Build history of the part. All positions in model axes, mm. A direction names the side the tool comes from. Round coordinates to 2 decimals unless told otherwise and drop trailing zeros. Loops run counter-clockwise (first coordinate to the right, second up) from the corner with the lowest first, then second, coordinate; pieces in that order, holes last. Notation, with made-up numbers: M 82,6 L 103,6 A27 ccw 103,38 Z; hole C 32.5,18.5 d7. An arc over 180 degrees is marked long. One line per item, written item: value.
Autodesk Inventor part; units mm, degrees
ref_plane "YZ Plane" through (0, 0, 0) normal (1, 0, 0) x (0, 1, 0)
ref_plane "XZ Plane" through (0, 0, 0) normal (0, 1, 0) x (-1, 0, 0)
ref_plane "XY Plane" through (0, 0, 0) normal (0, 0, 1) x (1, 0, 0)
sketch "Sketch1" plane through (0, 0, 0) normal (0, 1, 0) x (-1, 0, 0)
  line L0 (0, 0) -> (23.6236, 0) construction
  line L1 (0, 0) -> (0, -20.0966) construction
  arc A0 (-8, 0) -> (8, 0) centre (0, 0) ccw
  arc A1 (-2.9468, -7.4375) -> (2.9468, -7.4375) centre (0, -8) ccw
  line L2 (0, -11) -> (-8.5189, -11) construction
  circle A2 centre (0, -8) radius 1.35
  line L3 (-8, 0) -> (8, 0)
  arc A3 (8, 0) -> (-8, 0) centre (0, 0) ccw
  arc A4 (2.9468, 7.4375) -> (-2.9468, 7.4375) centre (0, 8) ccw
  line L4 (0, 11) -> (-8.5189, 11) construction
  circle A5 centre (0, 8) radius 1.35
  dimension "d0" = 16
  dimension "d1" = 22
  dimension "d2" = 6
  dimension "d3" = 2.7
extrude "Extrusion1" add sketch "Sketch1" along normal blind 8
extrude "Extrusion2" cut sketch "Sketch1" against normal blind 7 from surface at 8 contours A2 A0 | A0 A2 | A5 A3 | A3 A5
extrude "Extrusion3" add sketch "Sketch1" against normal blind 3.5 contours L3 A0 A2 | A3 A5 L3 | A2 A0 | A3 A5 picked at (0, -7.5415) picked at (0, 7.5415)
chamfer "Chamfer1" distance 1 angle 45 1 edges at (2.9468, -3.5, 7.4375)
properties part number "caster_body"
Item 1: Slice it at B-B, the plane y = 4.25. Give the cut face in (x, z), and give its area (3 significant figures).
Check values:
outline: M -2.95,-7.44 A3 ccw long 2.95,-7.44 A8 ccw 2.95,7.44 A3 ccw long -2.95,7.44 A8 ccw Z; hole C 0,-8 d2.7; hole C 0,8 d2.7
area: 220 mm2
Item 2: Wall check: line 1 along X through (y, z) = (6.25, -8); line 2 along Z through (x, y) = (0.75, 2.25); line 3 along Y through (x, z) = (-1.5, -7.75). Give the ranges that are in metal, low to high.
Check values:
line 1: x = -3 to -1.35, 1.35 to 3
line 2: z = -10.9 to -9.12, -6.88 to 6.88, 9.12 to 10.9
line 3: y = -2.61 to 8
Item 3: Which spindle directions (+Z, -Z, +X, -X, +Y, -Y) get a long thin tool onto all of the face, cutting with end or side? Do faces 1 (the face through (0, -3.5, 0)), 2 (the face through (0, 1, 8)). Say none if no direction does.
Check values:
face 1: +Z, -Z, +X, -X, -Y
face 2: +Y
Item 4: Slice it at C-C, the plane y = -1.75. Give the cut face in (x, z), and give its area (3 significant figures).
Check values:
outline: C 0,0 d16
area: 201 mm2
Item 5: Pull direction X, two halves, no side cores. Call faces 3 (the face through (0, 4, -11)), 4 (the face through (0, 8, 0)), 5 (the face through (0.176, 4.549, -6.661)): pulls with the +X half, pulls with the -X half, needs draft (parallel to the pull), parting line crosses it, or undercut.
Check values:
face 3: parting line crosses it
face 4: needs draft
face 5: undercut
Item 6: Slice it at A-A, the plane x = 0. Give the cut face in (y, z).
Check values:
outline: M -3.5,-7 L -2.5,-8 L 0,-8 L 0,-11 L 8,-11 L 8,-9.35 L 1,-9.35 L 1,-6.65 L 8,-6.65 L 8,6.65 L 1,6.65 L 1,9.35 L 8,9.35 L 8,11 L 0,11 L 0,8 L -2.5,8 L -3.5,7 Z
Item 7: Drop flat-ended pins along their axis: P1, Ø1, axis at x = -1.5, y = 2, coming from the +Z side; P2, Ø1.1, axis at x = 1, z = 9, coming from the -Y side; P3, Ø4, axis at y = -0.5, z = -4.5, coming from the -X side. Give the stop position or say it passes through.
Check values:
P1: stops at z = 10.83
P2: stops at y = 0
P3: stops at x = -7.6
